Read the model definition and answer for the solid it produces. Units are mm, in the model's axes. A direction names the side the tool comes from. Give positions to 0.01 mm unless a question says otherwise; leave off trailing zeros. Order: outer loops, then holes, each group sorted by start corner. A loop starts at its lowest first (then second) coordinate and runs counter-clockwise, first axis right, second up. Notation, with made-up numbers: (-9, 60.25) - (43, 60.25) arc R29 ccw to (43, 95.25) - close; hole circle Ø6 at (61.25, 9). An arc over 180 degrees is marked (long way). Use a Markdown table: item, result. Add a question column.
1. Consider L1, parallel to Y at x = -6.75, z = 0; L2, parallel to Y at x = 8, z = -3; L3, parallel to X at y = 16.5, z = 0. Determine where each line is inside the solid, lowest interval first.
2. Which of the six approach directions +Z, -Z, +X, -X, +Y, -Y give full straight-line access (tool end or side, diameter ignored) to faces 1 (the flat face through (-18, 14, 0)), 2 (the cylindrical face through (-19, 7, -4)), 3 (the flat face through (15, 14, 0))?
3. A cutting plane is placed at A-A on x = -5. Determine the outline of the cut face in (y, z).
4. A cutting plane is placed at B-B on y = 7. Determine the outline of the cut face in (x, z).
5. For a pull along Z with two mould halves and no side action, classify faces 4 (the flat face through (0, 16, 0)), 5 (the flat face through (-0.3, 10.4, -2)), 6 (the flat face through (-10, 19.9, -2.3)) as released by +Z, released by -Z, zero draft, split by the parting line, or undercut.
6. Flat-ended cylindrical pins translate along their axes: P1, Ø1.5, axis at x = -0.5, z = 0.5, coming from the +Y side; P2, Ø1.5, axis at y = 19, z = -1.5, coming from the +X side; P3, Ø3, axis at x = -18, z = -1, coming from the +Y side. Find the tip coordinate at first contact, or state that the pin passes through.
7. A cutting plane is placed at C-C on z = -3.5. Determine the outline of the cut face in (x, y).
8. A cutting plane is placed at D-D on x = 0. Determine the outline of the cut face in (y, z), and give its area (3 significant figures).
Autodesk Inventor part; units mm, degrees
ref_plane "YZ Plane" through (0, 0, 0) normal (1, 0, 0) x (0, 1, 0)
ref_plane "XZ Plane" through (0, 0, 0) normal (0, 1, 0) x (-1, 0, 0)
ref_plane "XY Plane" through (0, 0, 0) normal (0, 0, 1) x (1, 0, 0)
sketch "Sketch1" plane through (0, 0, 0) normal (0, 0, 1) x (1, 0, 0)
  line L0 (-25, 14) -> (-10, 14)
  line L1 (-10, 14) -> (-10, 26)
  line L2 (-10, 26) -> (5, 26)
  line L3 (5, 26) -> (5, 14)
  line L4 (5, 14) -> (25, 14)
  line L5 (25, 14) -> (25, 0)
  line L6 (25, 0) -> (-25, 0)
  line L7 (-25, 0) -> (-25, 14)
  line L8 (-16, 7) -> (16, 7) construction
  line L9 (-16, 4) -> (16, 4)
  line L10 (16, 10) -> (-16, 10)
  arc A0 (-16, 10) -> (-16, 4) centre (-16, 7) ccw
  arc A1 (16, 4) -> (16, 10) centre (16, 7) ccw
  line L11 (25, 12) -> (-25, 12)
  line L12 (-25, 2) -> (25, 2)
  point P0 (0, 0)
  point P1 (0, 0)
  point P2 (0, 7)
  point P3 (0, 26)
  point P4 (-10, 20)
  dimension "d0" = 26
  dimension "d1" = 14
  dimension "d2" = 50
  dimension "d3" = 15
  dimension "d4" = 15
  dimension "d7" = 32
  dimension "d8" = 6
  dimension "d9" = 10
extrude "Extrusion1" add sketch "Sketch1" along normal mid plane 10 contours L0 L1 L2 L3 L4 L5 L11 L7 | L11 L5 L12 L7 | L12 L5 L6 L7 | A0 L10 A1 L9
extrude "Extrusion2" cut sketch "Sketch1" along normal blind 5 and the other way blind 2 contours L11 L5 L12 L7
extrude "Extrusion3" cut sketch "Sketch1" along normal through all both and the other way through all contours A0 L10 A1 L9
hole "Hole1" at (0, 26, 0) direction (0, -1, 0) diameter 5 depth 10
hole "Hole2" at (-10, 20, 0) direction (1, 0, 0) diameter 3.6881 end up to surface
chamfer "Chamfer1" distance 0.1 angle 45 10 edges at (-10, 20, -1.8441) (0, 26, -2.5) (0, 4, -2) (19, 7, -2) (0, 10, -2) (-19, 7, -2) (0, 4, -5) (19, 7, -5) (0, 10, -5) (-19, 7, -5)
properties part number "Crosshead"
Output values:
| question | item | result |
|---|---|---|
| 1 | L1 | 0 to 2, 12 to 18.16, 21.84 to 26 |
| 1 | L2 | 0 to 4, 10 to 14 |
| 1 | L3 | -10 to -2.5, 2.5 to 5 |
| 2 | face 1 | +Z, -Z, -X, +Y |
| 2 | face 2 | +Z, -Z |
| 2 | face 3 | +Z, -Z, +X, +Y |
| 3 | outline | (0, -5) - (3.9, -5) - (4, -4.9) - (4, -2.1) - (3.9, -2) - (2, -2) - (2, 5) - (0, 5) - close; (10, -4.9) - (10.1, -5) - (26, -5) - (26, 5) - (12, 5) - (12, -2) - (10.1, -2) - (10, -2.1) - close; hole circle Ø3.69 at (20, 0) |
| 4 | outline | (-25, -5) - (-19.1, -5) - (-19, -4.9) - (-19, -2.1) - (-19.1, -2) - (-25, -2) - close; (19, -4.9) - (19.1, -5) - (25, -5) - (25, -2) - (19.1, -2) - (19, -2.1) - close |
| 5 | face 4 | undercut |
| 5 | face 5 | released by +Z |
| 5 | face 6 | zero draft |
| 6 | P1 | y = 16 |
| 6 | P2 | x = 5 |
| 6 | P3 | y = 14 |
| 7 | outline | (-25, 0) - (25, 0) - (25, 14) - (5, 14) - (5, 26) - (-10, 26) - (-10, 14) - (-25, 14) - close; hole (-16, 4) - (16, 4) arc R3 ccw to (16, 10) - (-16, 10) arc R3 ccw to start |
| 8 | outline | (0, -5) - (3.9, -5) - (4, -4.9) - (4, -2.1) - (3.9, -2) - (2, -2) - (2, 5) - (0, 5) - close; (10, -4.9) - (10.1, -5) - (26, -5) - (26, -2.6) - (25.9, -2.5) - (16, -2.5) - (16, 2.5) - (25.9, 2.5) - (26, 2.6) - (26, 5) - (12, 5) - (12, -2) - (10.1, -2) - (10, -2.1) - close |
| 8 | area | 122 mm² |
